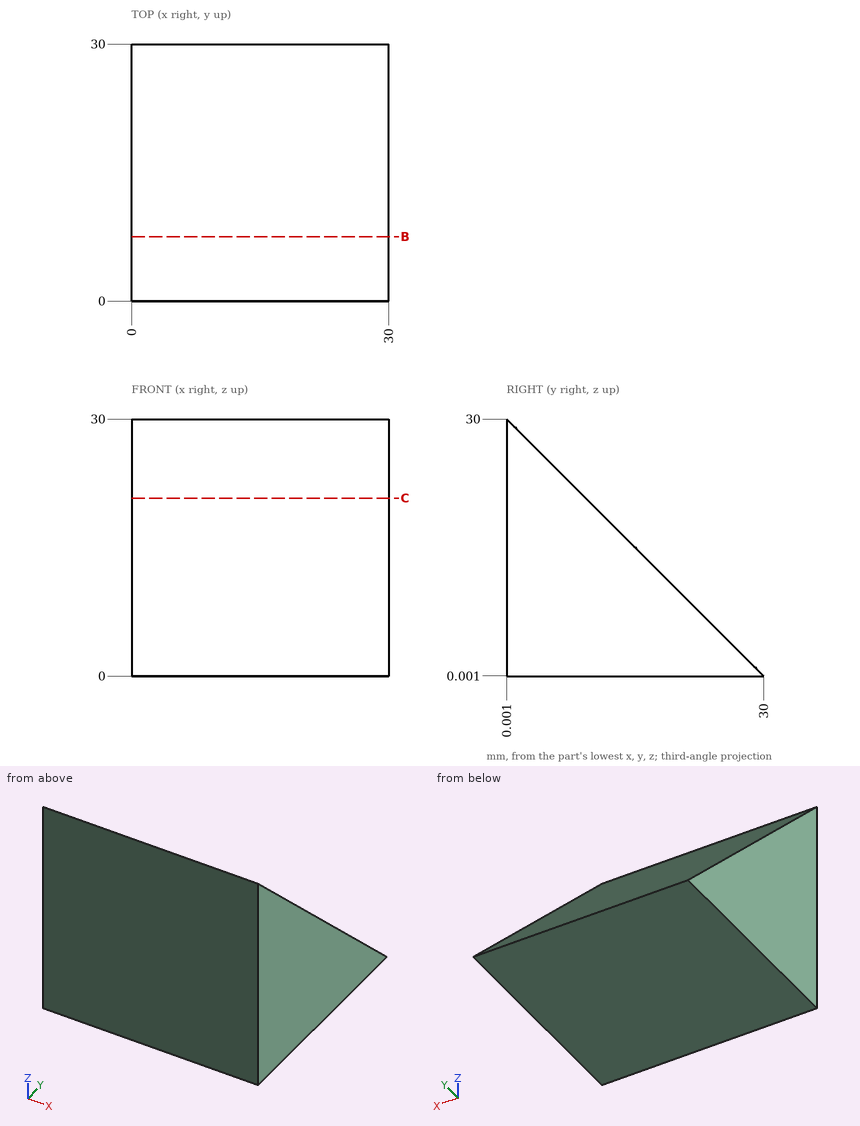
For this review, use the dimensioned drawing (mm, ordinates from the lowest corner) and the shaded views. Give positions to 0.01 mm unless a question says otherwise; leave off trailing zeros. Order: outer loops, then holes, each group sorted by start corner. A loop starts at its lowest first (then second) coordinate and runs counter-clockwise, first axis right, second up.
1. Add section B-B, the plane y = 7.5. State the section outline as (x, z) points.
Solution:
outline: (0, 0) - (30, 0) - (30, 22.5) - (0, 22.5) - close
2. Add section C-C, the plane z = 20.75. State the section outline as (x, y) points.
Solution:
outline: (0, 0) - (30, 0) - (30, 9.25) - (0, 9.25) - close
3. To check wall thickness, follow L1, parallel to Y at x = 9.25, z = 25.75; L2, parallel to Z at x = 23.5, y = 18; L3, parallel to Z at x = 20, y = 24. State the ranges of each line that lie inside material, in increasing order.
Solution:
L1: y = 0 to 4.25
L2: z = 0 to 12
L3: z = 0 to 6
4. For pin 1 Ø2 at (x, z) = (4, 7) entering from +Y; pin 2 Ø1.5 at (x, y) = (23.5, 10.5) entering from +Z, all flat-tipped, find the tip position at first contact; note any pin that passes through.
Solution:
pin 1: stops at y = 24
pin 2: stops at z = 20.25
